Could you check a few things on this model? Use its own coordinates, in mm. Face numbers are marked on the shaded views. A direction names the side the tool comes from. Round coordinates to 2 decimals unless told otherwise and drop trailing zeros. Loops run counter-clockwise (first coordinate to the right, second up) from the corner with the lowest first, then second, coordinate; pieces in that order, holes last.
from build123d import *

# Parameters (mm, degrees)
F0_R     = 2.75
F1_DEPTH = 5
F2_R     = 3.5661431143
F2_R_2   = 2.75
F3_DEPTH = 0.75
F5_DEPTH = 2.5
F6_DEPTH = 25


with BuildPart() as f1:
    # F0 (on Top) → F1 (new body)
    with BuildSketch(Plane.XY):
        Polygon((3.4641016151, 6), (-3.4641016151, 6), (-6.9282032303, 0), (-3.4641016151, -6), (3.4641016151, -6), (6.9282032303, 0), align=None)
        Circle(F0_R, mode=Mode.SUBTRACT)
    extrude(amount=F1_DEPTH)

    # F2 (on face) → F3 (join)
    with BuildSketch(Plane.XY.offset(5)):
        Circle(F2_R)
        Circle(F2_R_2, mode=Mode.SUBTRACT)
    extrude(amount=F3_DEPTH)

    # F4 (on face) → F5 (cut)
    with BuildSketch(Plane.XY.offset(5)):
        Polygon((-2.1890449113, 5.4928889455), (-3.906649748, 4.4682750548), (2.0444942813, -5.5078865623), (3.7620991179, -4.4832726717), align=None)
    extrude(amount=-F5_DEPTH, mode=Mode.SUBTRACT)

    # F6 (cut): faces of the model
    f6_faces = [f1.faces().sort_by_distance(p)[0] for p in [
        (-1.6478181141, 2.6289073274, 5),
        (1.5304323639, -2.698932206, 5),
        (-1.6478181141, 2.6289073274, 5),
        (1.5304323639, -2.698932206, 5),
    ]]
    extrude(f6_faces, amount=-F6_DEPTH, mode=Mode.SUBTRACT)


solid = f1.part
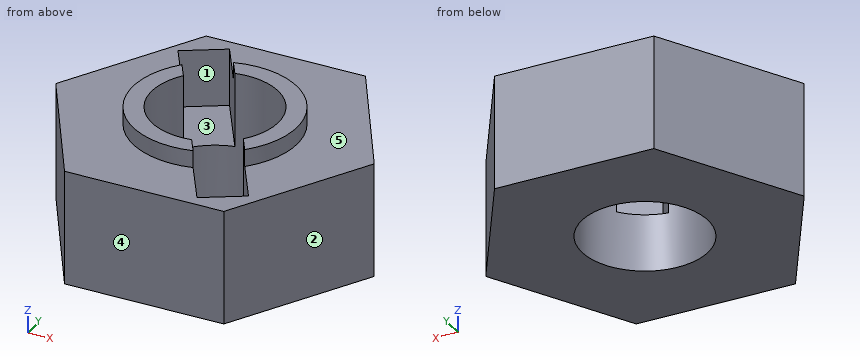
Item 1: If I drill on line 1 along Y through (x, z) = (0, 1.4); line 2 along Z through (x, y) = (-5.75, 0.5); line 3 along X through (y, z) = (2.5, 1.85), over which ranges is the centre line in solid material (lowest first)?
Results list:
line 1: y = -6 to -2.75, 2.75 to 6
line 2: z = 0 to 5
line 3: x = -5.48 to -1.15, 1.15 to 5.48
Item 2: If we section it at B-B, the plane z = 3.75: Please give me the cut outline in (x, y), then the cut area to 3 significant figures.
Results list:
outline: (-6.93, 0) - (-3.46, -6) - (3.46, -6) - (6.93, 0) - (3.46, 6) - (-3.46, 6) - close; hole (-3.91, 4.47) - (-2.21, 1.63) arc R2.75 ccw to (0.38, -2.72) - (2.04, -5.51) - (3.76, -4.48) - (2.13, -1.74) arc R2.75 ccw to (-0.52, 2.7) - (-2.19, 5.49) - close
area: 88.5 mm2
Item 3: For the marked faces 1 and 2, which set-ups out of +Z, -Z, +X, -X, +Y, -Y let a thin tool reach every point of the face, with its end or its side?
Results list:
face 1: +Z
face 2: +Z, -Z, +X, -Y
Item 4: If we section it at D-D, the plane z = 1.75: Please give me the cut outline in (x, y).
Results list:
outline: (-6.93, 0) - (-3.46, -6) - (3.46, -6) - (6.93, 0) - (3.46, 6) - (-3.46, 6) - close; hole circle Ø5.5 at (0, 0)
Item 5: If we section it at A-A, the plane x = 0: Please give me the cut outline in (y, z).
Results list:
outline: (-6, 0) - (-2.75, 0) - (-2.75, 5.75) - (-3.57, 5.75) - (-3.57, 5) - (-6, 5) - close; (2.75, 0) - (6, 0) - (6, 5) - (3.57, 5) - (3.57, 5.75) - (2.75, 5.75) - close
Item 6: If we section it at C-C, the plane y = 5.25: Please give me the cut outline in (x, z), then the cut area to 3 significant figures.
Results list:
outline: (-3.9, 0) - (3.9, 0) - (3.9, 5) - (-2.04, 5) - (-2.04, 2.5) - (-2.6, 2.5) - (-2.6, 5) - (-3.9, 5) - close
area: 37.6 mm2
Item 7: We'd pull the mould along Y, two halves only. Please class the marked faces 3, 4 and 5: released by +Y, released by -Y, zero draft, split by the parting line, or undercut.
Results list:
face 3: undercut
face 4: released by -Y
face 5: zero draft
Item 8: Will these pins go through, and if not, where does the flat tip stop? pin 1 (2 mm diameter, centred on x = 2.5, y = 4, fed in from +Z); pin 2 (3 mm diameter, centred on y = 3.5, z = 1, fed in from +X).
Results list:
pin 1: stops at z = 5
pin 2: stops at x = 5.77
